Geometry: final body of the model. Coordinates: model frame, mm. A direction names the side the tool comes from. Round coordinates to 2 decimals unless told otherwise and drop trailing zeros. Write each loop counter-clockwise with the first axis right and the second up, starting at its lowest first coordinate (ties: lowest second). Pieces come first, ordered by that corner, then holes. Notation, with made-up numbers: (75, 81.25) -> (132, 81.25) arc R32 ccw to (132, 119.25) -> close; hole circle Ø7 at (-4.75, 56). An arc over 180 degrees is marked (long way). One line per item, written item: value. Start each with the question number.
from build123d import *

# Parameters (mm, degrees)
SKETCH1_R           = 7.874
SKETCH1_W           = 25.4
SKETCH1_H           = 80.9625
BOSS_EXTRUDE1_DEPTH = 12.7
SKETCH2_W           = 20
SKETCH2_H           = 41
CUT_EXTRUDE1_DEPTH  = 13.7
SKETCH3_W           = 20
SKETCH3_H           = 41
CUT_EXTRUDE2_DEPTH  = 13.7


with BuildPart() as part:
    # Sketch1 → Boss-Extrude1 (new body)
    with BuildSketch(Plane(origin=(0, 0, 0), x_dir=(1, 0, 0), z_dir=(0, 1, 0))):
        Polygon((0, 241.3), (0, 0), (25.4, 0), (101.6, 0), (127, 0), (127, 241.3), align=None)
        with Locations((63.5, 190.5)):
            Circle(SKETCH1_R, mode=Mode.SUBTRACT)
        with Locations((12.7, -40.48125)):
            Rectangle(SKETCH1_W, SKETCH1_H)
        with Locations((114.3, -40.48125)):
            Rectangle(SKETCH1_W, SKETCH1_H)
    extrude(amount=BOSS_EXTRUDE1_DEPTH)

    # Sketch2 → Cut-Extrude1 (cut, through all)
    with BuildSketch(Plane.XZ):
        with Locations((104.3, -175.05319538)):
            Rectangle(SKETCH2_W, SKETCH2_H)
    extrude(amount=-CUT_EXTRUDE1_DEPTH, mode=Mode.SUBTRACT)

    # Sketch3 → Cut-Extrude2 (cut, through all)
    with BuildSketch(Plane(origin=(0, 0, 0), x_dir=(-1, 0, 0), z_dir=(0, -1, 0))):
        with Locations((-22.7, 79.2375)):
            Rectangle(SKETCH3_W, SKETCH3_H)
    extrude(amount=-CUT_EXTRUDE2_DEPTH, mode=Mode.SUBTRACT)


solid = part.part
(1) Section query A-A (z = 59). Output: boundary loops of the cut face in (x, y).
(2) Line query: probe 1 along X at (y, z) = (7, -190.5); probe 2 along X at (y, z) = (7, 38); probe 3 along Z at (x, y) = (29, 1). Output: solid intervals per line, ascending.
(3) Section query D-D (y = 6.25). Output: boundary loops of the cut face in (x, z).
(4) Pull-direction query (X, two-part tool) for faces 4 (the face through (0, 6, -82)), 5 (the face through (63, 12.7, -82)), 6 (the face through (104, 6, -195.553)); classes: pulls with the +X half, pulls with the -X half, needs draft (parallel to the pull), parting line crosses it, or undercut.
(5) Section query C-C (z = -190.5). Output: boundary loops of the cut face in (x, y), and give its area (3 significant figures).
(6) Section query B-B (x = 63.5). Output: boundary loops of the cut face in (y, z), and give its area (3 significant figures).
(7) Pin query (flat end, axial travel): pin 1 (4 mm diameter, centred on x = 72, y = 10.5, fed in from +Z). Return the tip coordinate at first contact, or that it passes through.
(8) Set-up query: faces 1 (the face through (114.3, 6, -175)), 2 (the face through (63, 6, 0)), 3 (the face through (64, 6, -241.3)). Return all of +Z, -Z, +X, -X, +Y, -Y with unobstructed straight access to the full face (end or side cutting, diameter ignored); none if empty.
Results list:
1. outline: (0, 0) -> (25.4, 0) -> (25.4, 12.7) -> (0, 12.7) -> close; (101.6, 0) -> (127, 0) -> (127, 12.7) -> (101.6, 12.7) -> close
2. probe 1: x = 0 to 55.63, 71.37 to 94.3, 114.3 to 127
2. probe 2: x = 0 to 25.4, 101.6 to 127
2. probe 3: z = -241.3 to -99.74, -58.74 to 0
3. outline: (0, -241.3) -> (127, -241.3) -> (127, 80.96) -> (101.6, 80.96) -> (101.6, 0) -> (25.4, 0) -> (25.4, 80.96) -> (0, 80.96) -> close; hole (12.7, -99.74) -> (32.7, -99.74) -> (32.7, -58.74) -> (12.7, -58.74) -> close; hole circle Ø15.75 at (63.5, -190.5); hole (94.3, -195.55) -> (114.3, -195.55) -> (114.3, -154.55) -> (94.3, -154.55) -> close
4. face 4: pulls with the -X half
4. face 5: needs draft
4. face 6: undercut
5. outline: (0, 0) -> (55.63, 0) -> (55.63, 12.7) -> (0, 12.7) -> close; (71.37, 0) -> (94.3, 0) -> (94.3, 12.7) -> (71.37, 12.7) -> close; (114.3, 0) -> (127, 0) -> (127, 12.7) -> (114.3, 12.7) -> close
5. area: 1,160 mm^2
6. outline: (0, -241.3) -> (12.7, -241.3) -> (12.7, -198.37) -> (0, -198.37) -> close; (0, -182.63) -> (12.7, -182.63) -> (12.7, 0) -> (0, 0) -> close
6. area: 2,860 mm^2
7. pin 1: stops at z = 0
8. face 1: +Y, -Y
8. face 2: +Z, +Y, -Y
8. face 3: -Z, +X, -X, +Y, -Y
